Here's the drawing with two shaded views (mm, measured from the low corner). I have some questions. Round coordinates to 2 decimals unless told otherwise and drop trailing zeros. Loops run counter-clockwise (first coordinate to the right, second up) from the corner with the lowest first, then second, coordinate; pieces in that order, holes last. Notation, with made-up numbers: M 10.25,19.5 L 65.25,19.5 A23 ccw 65.25,30.5 Z; hole C 40,20.5 d7. An arc over 180 degrees is marked long. Answer as a JSON object with one key per item and string values.
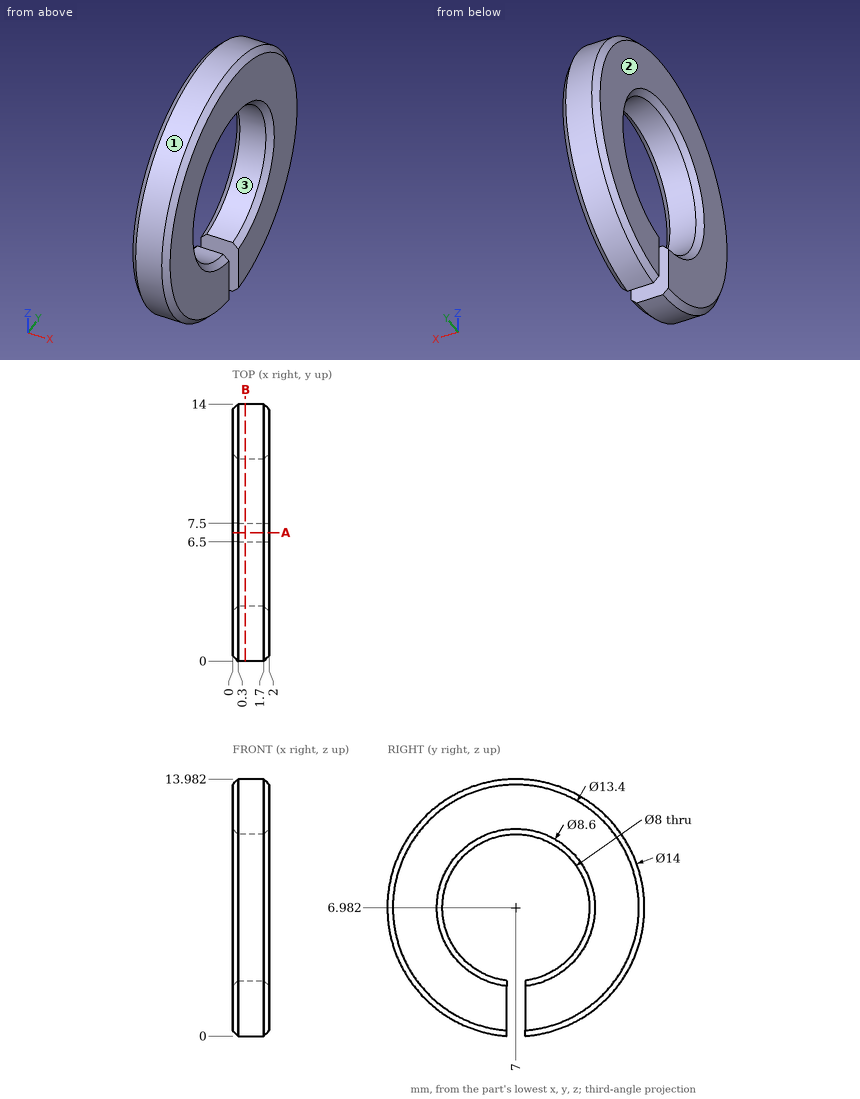
Item 1: I want a section at B-B on x = 0.7. List the corners of the cut face in (y, z) for me, plus the area to 3 significant figures.
Solution:
{"outline": "M 6.5,0 L 6.5,3.01 A4 cw long 7.5,3.01 L 7.5,0 A7 ccw long Z", "area": "101 mm2"}
Item 2: We'd pull the mould along Y, two halves only. Please class the marked faces 1, 2 and 3: +Y half, -Y half, draft (parallel to the pull), parting line (faces both ways), or undercut.
Solution:
{"face 1": "parting line", "face 2": "draft", "face 3": "undercut"}
Item 3: I want a section at A-A on y = 7. List the corners of the cut face in (x, z) for me.
Solution:
{"outline": "M 0,11.28 L 0.3,10.98 L 1.7,10.98 L 2,11.28 L 2,13.68 L 1.7,13.98 L 0.3,13.98 L 0,13.68 Z"}
Item 4: If I drill on L1, parallel to Y at x = 0.8, z = 7; L2, parallel to Y at x = 1.6, z = 10.5; L3, parallel to Z at x = 1.55, y = 9.5 (1 decimal), over which ranges is the centre line in solid material (lowest first)? Write a range as from..to.
Solution:
{"L1": "y = 0..3, 11..14", "L2": "y = 0.95..5.1, 8.9..13.05", "L3": "z = 0.4..3.9, 10.1..13.5"}
Item 5: For P1, Ø1, axis at x = 1, y = 8.5, coming from the +Z side; P2, Ø7, axis at y = 7, z = 6.98, coming from the +X side; P3, Ø1, axis at x = 1, z = 1, coming from the -Y side, each with a flat end and sliding along its axis, tell me the tip position at first contact or that it passes through.
Solution:
{"P1": "stops at z = 13.91", "P2": "passes through", "P3": "stops at y = 2.65"}
